from build123d import *

# Parameters (mm, degrees)
SKETCH_1_R          = 2.5
EXTRUDE_1_DEPTH     = 45
SKETCH_2_R          = 4
EXTRUDE_2_DEPTH     = 3
CHAMFER_1_SIZE      = 1
SKETCH_3_W          = 1
SKETCH_3_H          = 8
CUT_EXTRUDE_1_DEPTH = 1.5


with BuildPart() as part:
    # Эскиз1 → Бобышка-Вытянуть1 (new body)
    with BuildSketch(Plane.XY):
        Circle(SKETCH_1_R)
    extrude(amount=EXTRUDE_1_DEPTH)

    # Эскиз2 → Бобышка-Вытянуть2 (add)
    with BuildSketch(Plane.XY.offset(45)):
        Circle(SKETCH_2_R)
    extrude(amount=-EXTRUDE_2_DEPTH)

    # Фаска1
    chamfer_1_edges = [part.edges().sort_by_distance(p)[0] for p in [
        (-2.5, 0, 0),
    ]]
    chamfer(chamfer_1_edges, length=CHAMFER_1_SIZE)

    # Эскиз3 → Вырез-Вытянуть1 (cut)
    with BuildSketch(Plane.XY.offset(45)):
        Rectangle(SKETCH_3_W, SKETCH_3_H)
    extrude(amount=-CUT_EXTRUDE_1_DEPTH, mode=Mode.SUBTRACT)


solid = part.part
The model under review builds one solid part; all positions refer to its coordinate system, in mm. A direction names the side the tool comes from. Coordinates: 2 decimals unless noted, no trailing zeros. Loops run counter-clockwise (first coordinate to the right, second up) from the corner with the lowest first, then second, coordinate; pieces in that order, holes last. Notation, with made-up numbers: M -33.75,45 L 10.25,45 A27 ccw 10.25,67 Z; hole C 70.25,75.5 d10. An arc over 180 degrees is marked long. Put each result on its own line as item: value. Start each with the question number.
Q1. Clearance check with flat-ended pins moving along their axes: pin 1 (1.5 mm diameter, centred on y = 0, z = 30.5, fed in from +X); pin 2 (1 mm diameter, centred on x = 1.5, z = 34.5, fed in from -Y); pin 3 (0.8 mm diameter, centred on y = -1, z = 44.5, fed in from +X). State where each tip first meets the part, or that it passes through.
Q2. Add section D-D (x = 3.25). Write out the cut boundary in (y, z), and give its area (3 significant figures).
Q3. For faces 1 (the cylindrical face through (-0.54, -2.44, 21.21)), 2 (the flat face through (-0.5, 0, 44)), 3 (the flat face through (2, 0, 45)), list the 3-axis set-ups (+Z, -Z, +X, -X, +Y, -Y) from which the entire face can be reached by the end or side of a thin tool; tool diameter is ignored.
Q4. The part is to be moulded in two halves that separate along X. For faces 4 (the flat face through (0, 0, 43.5)), 5 (the flat face through (2, 2, 42)), 6 (the cylindrical face through (-0.867, -3.905, 43.521)), 7 (the flat face through (0.5, 0, 44)), say which applies: +X half, -X half, draft (parallel to the pull), parting line (faces both ways), or undercut.
Q5. Add section B-B (y = 0). Write out the cut boundary in (x, z), and give its area (4 significant figures).
Q6. Add section C-C (z = 23). Write out the cut boundary in (x, y).
Q7. Wall thickness on line 1 (Z direction, x = -3.5, y = 0.25); line 2 (Y direction, x = 0, z = 29): over which ranges is each line inside the solid? List them lowest first.
Q8. Add section A-A (x = 0). Write out the cut boundary in (y, z), and give its area (3 significant figures).
Answers:
1. pin 1: stops at x = 2.5
1. pin 2: stops at y = -2.29
1. pin 3: stops at x = 3.95
2. outline: M -2.33,42 L 2.33,42 L 2.33,45 L -2.33,45 Z
2. area: 14.0 mm^2
3. face 1: -Z
3. face 2: +Z, +Y, -Y
3. face 3: +Z, +X, -X, +Y, -Y
4. face 4: undercut
4. face 5: draft
4. face 6: parting line
4. face 7: undercut
5. outline: M -4,42 L -2.5,42 L -2.5,1 L -1.5,0 L 1.5,0 L 2.5,1 L 2.5,42 L 4,42 L 4,45 L 0.5,45 L 0.5,43.5 L -0.5,43.5 L -0.5,45 L -4,45 Z
5. area: 231.5 mm^2
6. outline: C 0,0 d5
7. line 1: z = 42 to 45
7. line 2: y = -2.5 to 2.5
8. outline: M -4,42 L -2.5,42 L -2.5,1 L -1.5,0 L 1.5,0 L 2.5,1 L 2.5,42 L 4,42 L 4,43.5 L -4,43.5 Z
8. area: 221 mm^2
